Part model, mm, in its own coordinate system. Round coordinates to 2 decimals unless told otherwise and drop trailing zeros. Write each loop counter-clockwise with the first axis right and the second up, starting at its lowest first coordinate (ties: lowest second). Pieces come first, ordered by that corner, then holes. Notation, with made-up numbers: M 22.5,76.5 L 53.5,76.5 A11 cw 53.5,83.5 Z; hole C 87,-33 d2. An arc over 180 degrees is marked long. Use a Markdown table: item, result. Add a question column.
1) Drop flat-ended pins along their axis: P1, Ø1.5, axis at y = -55, z = 1, coming from the -X side; P2, Ø2.5, axis at x = -41, y = -58.3, coming from the -Z side; P3, Ø1.5, axis at y = -56, z = 1.5, coming from the +X side; P4, Ø1.5, axis at x = 6.5, z = 2, coming from the +Y side. Give the stop position or say it passes through.
2) Slice it at C-C on x = 41. Write the cut outline in (y, z), plus the area to 3 significant figures.
3) Slice it at B-B on y = -54.75. Write the cut outline in (x, z).
4) Slice it at A-A on z = 1.7. Write the cut outline in (x, y).
5) Wall check: probe 1 along X at (y, z) = (-55.75, 0.6); probe 2 along Y at (x, z) = (41, 1.35); probe 3 along Y at (x, z) = (-10.5, 2.8). Give the ranges that are in metal, low to high.
6) Slice it at D-D on x = -14. Write the cut outline in (y, z), plus the area to 3 significant figures.
```python
from build123d import *

# Parameters (mm, degrees)
F_01_REMOVABLE_UPPER_CROSSBAR_DEPTH = 3
S02_FASTENING_LUG_0_R               = 1.7
F_02_FASTENING_LUG_0_DEPTH          = 3
S03_FASTENING_LUG_1_R               = 1.7
F_03_FASTENING_LUG_1_DEPTH          = 3


with BuildPart() as part:
    # S01 - Removable upper crossbar → 01 - Removable upper crossbar (new body)
    with BuildSketch(Plane.XY):
        with BuildLine():
            Line((-43.5, -53.7), (43.5, -53.7))
            ThreePointArc((43.5, -53.7), (45.267766953, -52.967766953), (46, -51.2))
            Line((46, -51.2), (46, -49.2))
            ThreePointArc((46, -49.2), (45.267766953, -47.432233047), (43.5, -46.7))
            Line((43.5, -46.7), (-43.5, -46.7))
            ThreePointArc((-43.5, -46.7), (-45.267766953, -47.432233047), (-46, -49.2))
            Line((-46, -49.2), (-46, -51.2))
            ThreePointArc((-46, -51.2), (-45.267766953, -52.967766953), (-43.5, -53.7))
        make_face()
    extrude(amount=F_01_REMOVABLE_UPPER_CROSSBAR_DEPTH)

    # S02 - Fastening lug 0 → 02 - Fastening lug 0 (add)
    with BuildSketch(Plane.XY):
        with BuildLine():
            Line((-45.5, -58.3), (-45.5, -50.2))
            ThreePointArc((-45.5, -50.2), (-41, -45.7), (-36.5, -50.2))
            Line((-36.5, -50.2), (-36.5, -58.3))
            ThreePointArc((-36.5, -58.3), (-41, -62.8), (-45.5, -58.3))
        make_face()
        with Locations((-41, -58.3)):
            Circle(S02_FASTENING_LUG_0_R, mode=Mode.SUBTRACT)
    extrude(amount=F_02_FASTENING_LUG_0_DEPTH)

    # S03 - Fastening lug 1 → 03 - Fastening lug 1 (add)
    with BuildSketch(Plane.XY):
        with BuildLine():
            Line((36.5, -58.3), (36.5, -50.2))
            ThreePointArc((36.5, -50.2), (41, -45.7), (45.5, -50.2))
            Line((45.5, -50.2), (45.5, -58.3))
            ThreePointArc((45.5, -58.3), (41, -62.8), (36.5, -58.3))
        make_face()
        with Locations((41, -58.3)):
            Circle(S03_FASTENING_LUG_1_R, mode=Mode.SUBTRACT)
    extrude(amount=F_03_FASTENING_LUG_1_DEPTH)


solid = part.part
```
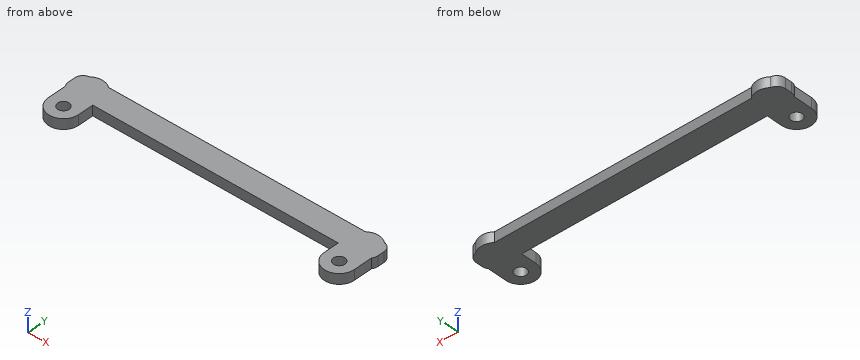
Entries:
| question | item | result |
|---|---|---|
| 1 | P1 | stops at x = -45.5 |
| 1 | P2 | passes through |
| 1 | P3 | stops at x = 45.5 |
| 1 | P4 | stops at y = -46.7 |
| 2 | outline | M -62.8,0 L -60,0 L -60,3 L -62.8,3 Z; M -56.6,0 L -45.7,0 L -45.7,3 L -56.6,3 Z |
| 2 | area | 41.1 mm^2 |
| 3 | outline | M -45.5,0 L -36.5,0 L -36.5,3 L -45.5,3 Z; M 36.5,0 L 45.5,0 L 45.5,3 L 36.5,3 Z |
| 4 | outline | M -46,-51.2 A2.5 ccw -45.5,-52.7 L -45.5,-58.3 A4.5 ccw -36.5,-58.3 L -36.5,-53.7 L 36.5,-53.7 L 36.5,-58.3 A4.5 ccw 45.5,-58.3 L 45.5,-52.7 A2.5 ccw 46,-51.2 L 46,-49.2 A2.5 ccw 43.86,-46.73 A4.5 ccw 38.17,-46.7 L -38.17,-46.7 A4.5 ccw -43.86,-46.73 A2.5 ccw -46,-49.2 Z; hole C -41,-58.3 d3.4; hole C 41,-58.3 d3.4 |
| 5 | probe 1 | x = -45.5 to -36.5, 36.5 to 45.5 |
| 5 | probe 2 | y = -62.8 to -60, -56.6 to -45.7 |
| 5 | probe 3 | y = -53.7 to -46.7 |
| 6 | outline | M -53.7,0 L -46.7,0 L -46.7,3 L -53.7,3 Z |
| 6 | area | 21.0 mm^2 |
